The listing builds one solid part. Answer for the finished solid, in the listing's coordinates (mm). Coordinates: 2 decimals unless noted, no trailing zeros. Order: outer loops, then holes, each group sorted by start corner. A loop starts at its lowest first (then second) coordinate and runs counter-clockwise, first axis right, second up. Notation, with made-up numbers: (70, 46) -> (90, 46) arc R23 cw to (90, 56) -> close; hole circle Ø6 at (44.25, 60.25). An arc over 180 degrees is marked (long way). One line per question, with ' | ' between items.
from build123d import *

# Parameters (mm, degrees)
SKETCH1_W             = 25.4
SKETCH1_H             = 47
BOSS_EXTRUDE1_DEPTH   = 3.175
SKETCH2_R             = 4.5
CUT_EXTRUDE1_DEPTH    = 27.90019749
FILLET1_R             = 3.175
M4X0_7_TAPPED_HOLE1_D = 3.3


with BuildPart() as part:
    # Sketch1 → Boss-Extrude1 (new body)
    with BuildSketch(Plane.XY):
        Rectangle(SKETCH1_W, SKETCH1_H)
    extrude(amount=BOSS_EXTRUDE1_DEPTH)

    # Sketch2 → Cut-Extrude1 (cut, through all)
    with BuildSketch(Plane.XY.offset(3.175)):
        with Locations((0, 10.25)):
            Circle(SKETCH2_R)
    extrude(amount=-CUT_EXTRUDE1_DEPTH, mode=Mode.SUBTRACT)

    # Fillet1
    fillet1_edges = [part.edges().sort_by_distance(p)[0] for p in [
        (12.7, -23.5, 1.5875),
        (-12.7, -23.5, 1.5875),
        (-12.7, 23.5, 1.5875),
        (12.7, 23.5, 1.5875),
    ]]
    fillet(fillet1_edges, radius=FILLET1_R)

    # M4x0.7 Tapped Hole1 (through all)
    with Locations(Plane.XY.offset(3.175)):
        with Locations((-6.35, -16), (6.35, -16)):
            Hole(M4X0_7_TAPPED_HOLE1_D / 2)


solid = part.part
Item 1: Section A-A, the plane z = 0.8 is taken. Give the vertices of the cut face in (x, y) (3 decimals), plus the area to 3 significant figures.
Computed values:
outline: (-12.7, -20.325) arc R3.175 ccw to (-9.525, -23.5) -> (9.525, -23.5) arc R3.175 ccw to (12.7, -20.325) -> (12.7, 20.325) arc R3.175 ccw to (9.525, 23.5) -> (-9.525, 23.5) arc R3.175 ccw to (-12.7, 20.325) -> close; hole circle Ø3.3 at (-6.35, -16); hole circle Ø9 at (0, 10.25); hole circle Ø3.3 at (6.35, -16) | area: 1,100 mm^2
Item 2: Determine the mould class of faces 1 (the face through (11.75, -22.59, 1.61)), 2 (the face through (-0.59, 14.71, 1.61)), 3 (the face through (0, 0, 0)), 4 (the face through (4.776, -15.504, 1.565)) for opening direction X: pulls with the +X half, pulls with the -X half, needs draft (parallel to the pull), parting line crosses it, or undercut.
Computed values:
face 1: pulls with the +X half | face 2: undercut | face 3: needs draft | face 4: undercut
Item 3: Find the intervals of material crossed by L1, parallel to Y at x = 6.35, z = 0.9; L2, parallel to Y at x = 0, z = 0.8; L3, parallel to X at y = -15, z = 2.65, in increasing order.
Computed values:
L1: y = -23.5 to -17.65, -14.35 to 23.5 | L2: y = -23.5 to 5.75, 14.75 to 23.5 | L3: x = -12.7 to -7.66, -5.04 to 5.04, 7.66 to 12.7
Item 4: Section B-B, the plane x = 0 is taken. Give the vertices of the cut face in (y, z) (3 decimals).
Computed values:
outline: (-23.5, 0) -> (5.75, 0) -> (5.75, 3.175) -> (-23.5, 3.175) -> close; (14.75, 0) -> (23.5, 0) -> (23.5, 3.175) -> (14.75, 3.175) -> close
Item 5: Section D-D, the plane y = -16 is taken. Give the vertices of the cut face in (x, z) (3 decimals).
Computed values:
outline: (-12.7, 0) -> (-8, 0) -> (-8, 3.175) -> (-12.7, 3.175) -> close; (-4.7, 0) -> (4.7, 0) -> (4.7, 3.175) -> (-4.7, 3.175) -> close; (8, 0) -> (12.7, 0) -> (12.7, 3.175) -> (8, 3.175) -> close
Item 6: Section C-C, the plane y = 10.25 is taken. Give the vertices of the cut face in (x, z) (3 decimals), plus the area to 3 significant figures.
Computed values:
outline: (-12.7, 0) -> (-4.5, 0) -> (-4.5, 3.175) -> (-12.7, 3.175) -> close; (4.5, 0) -> (12.7, 0) -> (12.7, 3.175) -> (4.5, 3.175) -> close | area: 52.1 mm^2
